Design review of the part built by this model. Coordinates are the model's own, in mm. Face numbers are marked on the shaded views. A direction names the side the tool comes from. Coordinates: 2 decimals unless noted, no trailing zeros. Write each loop counter-clockwise with the first axis right and the second up, starting at its lowest first coordinate (ties: lowest second). Pieces come first, ordered by that corner, then holes. Notation, with made-up numbers: M 2,61.25 L 7,61.25 A23 cw 7,93.25 Z; hole C 63,-16.75 d10. An arc over 180 degrees is marked long. Write item = value, one per line.
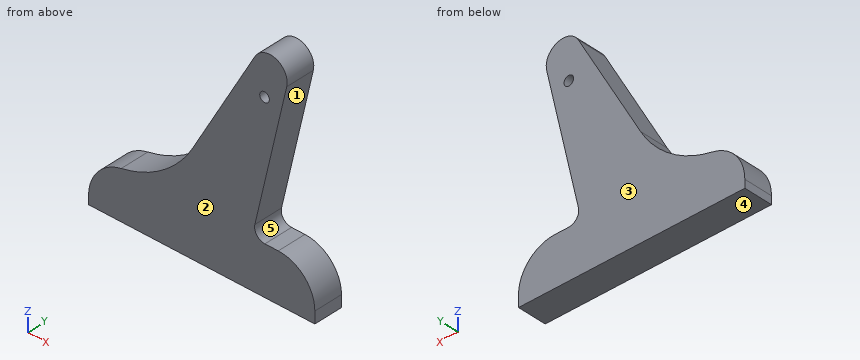
```python
from build123d import *

# Parameters (mm, degrees)
F0_R     = 1.27
F1_DEPTH = 7.62
F2_R     = 10.731179
F3_R     = 27.853237
F4_R     = 4.531262
F5_R     = 9.658061
F6_R     = 2.719813


with BuildPart() as f1:
    # F0 (on Front) → F1 (new body)
    with BuildSketch(Plane.XZ):
        Polygon((-31.954539, 12.834297), (-31.954539, 0), (0, 0), (27.812107, 0), (27.812107, 12.72366), (11.206285, 12.72366), (27.512231, 83.545011), (-12.00365, 12.834297), align=None)
        with Locations((14.526148, 47.354116)):
            Circle(F0_R, mode=Mode.SUBTRACT)
    extrude(amount=F1_DEPTH)

    # F2
    f2_edges = [f1.edges().sort_by_distance(p)[0] for p in [
        (-31.954539, -3.81, 12.834297),
    ]]
    fillet(f2_edges, radius=F2_R)

    # F3
    f3_edges = [f1.edges().sort_by_distance(p)[0] for p in [
        (-12.00365, -3.81, 12.834297),
    ]]
    fillet(f3_edges, radius=F3_R)

    # F4
    f4_edges = [f1.edges().sort_by_distance(p)[0] for p in [
        (27.512231, -3.81, 83.545011),
    ]]
    fillet(f4_edges, radius=F4_R)

    # F5
    f5_edges = [f1.edges().sort_by_distance(p)[0] for p in [
        (27.812107, -3.81, 12.72366),
    ]]
    fillet(f5_edges, radius=F5_R)

    # F6
    f6_edges = [f1.edges().sort_by_distance(p)[0] for p in [
        (11.206285, -3.81, 12.72366),
    ]]
    fillet(f6_edges, radius=F6_R)


solid = f1.part
```
Q1. Wall thickness on line 1 (X direction, y = -1.5, z = 46.5); line 2 (X direction, y = -2, z = 36); line 3 (Z direction, x = -7.5, y = -7): over which ranges is each line inside the solid? List them lowest first.
Check result:
line_1 = 6.81 to 13.59, 15.47 to 18.98
line_2 = 0.94 to 16.57
line_3 = 0 to 21.95
Q2. Consider section A-A, the plane z = 39.5. State the section outline as (x, y) points.
Check result:
outline = M 2.9,-7.62 L 17.37,-7.62 L 17.37,0 L 2.9,0 Z
Q3. Consider section B-B, the plane x = 8.5. State the section outline as (y, z) points.
Check result:
outline = M -7.62,0 L 0,0 L 0,49.52 L -7.62,49.52 Z
Q4. The part is to be moulded in two halves that separate along Z. For the marked faces 3, 4 and 5, say which applies: +Z half, -Z half, draft (parallel to the pull), parting line (faces both ways), or undercut.
Check result:
face_3 = draft
face_4 = -Z half
face_5 = undercut
Q5. Machinability: for the marked faces 1 and 2, which of the approach directions +Z, -Z, +X, -X, +Y, -Y give a long, thin tool a straight path to every point of the face, cutting with its end or side? Answer none if there is none.
Check result:
face_1 = +X, +Y, -Y
face_2 = +Z, -Z, +X, -X, -Y
Q6. For P1, Ø3, axis at x = 16.5, y = -4.5, coming from the +Z side; P2, Ø2, axis at x = 14.53, z = 47.35, coming from the -Y side; P3, Ø2, axis at y = -3, z = 23, coming from the -X side; P4, Ø1, axis at x = 19, y = -2.5, coming from the +Z side, all flat-tipped, find the tip position at first contact; note any pin that passes through.
Check result:
P1 = 58.13
P2 = through
P3 = -7.46
P4 = 57.36
